Input: part model. Units: mm. Frame: model coordinates. A direction names the side the tool comes from. Round coordinates to 2 decimals unless told otherwise and drop trailing zeros. Loops run counter-clockwise (first coordinate to the right, second up) from the corner with the lowest first, then second, coordinate; pieces in that order, holes last. Notation, with made-up numbers: M 66,-17.75 L 77,-17.75 A5 ccw 77,-12.75 Z; hole C -1.5,29.5 d5. An arc over 180 degrees is marked long. Return JSON: item names as keys, results as strings. Group by question number.
1) Mould query, pull axis X, two halves, no side actions, for faces 1 (the face through (-8.577, 2.348, -103.456)), 2 (the face through (-217, 4.762, -61)), 3 (the face through (0, 7, -48)). Classes: +X half, -X half, draft (parallel to the pull), parting line (faces both ways), or undercut.
2) Section A-A (z = -84.5). Output: boundary loops of the cut face in (x, y), plus the area to 3 significant figures.
3) Contact query for flat-ended pins moving along their axis: P1, Ø10, axis at x = -52.5, y = 7, coming from the +Z side; P2, Ø15, axis at x = -119, y = 34, coming from the -Z side; P3, Ø4.5, axis at x = -298, y = 7.5, coming from the -Z side; P4, Ø1, axis at x = -162, y = 12, coming from the -Z side. Output: stop coordinate, or through.
4) Access query for faces 4 (the face through (-219, 4.762, -9)), 5 (the face through (-219, 9.538, -40)), 6 (the face through (-431.8, 7, -44)), 7 (the face through (-423.43, 2.348, -103.654)). Directions: +Z, -Z, +X, -X, +Y, -Y. A direction counts if a zero-diameter tool reaches every point of the face in a straight line with its end or side. Return the directions, or none.
5) Section C-C (y = 20). Output: boundary loops of the cut face in (x, z), plus the area to 3 significant figures.
6) Section B-B (x = -78.5). Output: boundary loops of the cut face in (y, z), plus the area to 3 significant figures.
7) Material intervals for line 1 (Y direction, x = -396.5, z = -32.5); line 2 (Z direction, x = -53.5, y = 5.5); line 3 (Z direction, x = -121.5, y = 35), sorted ascending. Write a range as from..to.
8) Section D-D (z = -67). Output: boundary loops of the cut face in (x, y), plus the area to 3 significant figures.
from build123d import *

# Parameters (mm, degrees)
F1_DEPTH = 4.7625
F3_DEPTH = 431.8


with BuildPart() as f1:
    # F0 (on Front) → F1 (new body)
    with BuildSketch(Plane.XZ):
        with BuildLine():
            Line((0, 0), (-215.9, 0))
            Line((-215.9, 0), (-431.8, 0))
            Line((-431.8, 0), (-431.8, -112.7125))
            Line((-431.8, -112.7125), (-427.228, -112.7125))
            ThreePointArc((-427.228, -112.7125), (-423.326818, -103.5544), (-414.02, -100.022664))
            Line((-414.02, -100.022664), (-414.02, -91.132664))
            ThreePointArc((-414.02, -91.132664), (-398.8091, -80.428959), (-394.97, -62.23))
            Line((-394.97, -62.23), (-215.9, -62.23))
            Line((-215.9, -62.23), (-36.83, -62.23))
            ThreePointArc((-36.83, -62.23), (-32.9909, -80.428959), (-17.78, -91.132664))
            Line((-17.78, -91.132664), (-17.78, -100.022664))
            ThreePointArc((-17.78, -100.022664), (-8.473182, -103.5544), (-4.572, -112.7125))
            Line((-4.572, -112.7125), (0, -112.7125))
            Line((0, -112.7125), (0, 0))
        make_face()
    extrude(amount=-F1_DEPTH)

    # F2 (on face) → F3 (join, through all)
    with BuildSketch(Plane(origin=(-431.8, 0, 0), x_dir=(0, -1, 0), z_dir=(-1, 0, 0))):
        with BuildLine():
            Line((-4.7625, -55.88), (-4.7625, -17.78))
            Line((-4.7625, -17.78), (-42.3545, -17.78))
            ThreePointArc((-42.3545, -17.78), (-42.71371, -17.92879), (-42.8625, -18.288))
            Line((-42.8625, -18.288), (-42.8625, -22.0345))
            ThreePointArc((-42.8625, -22.0345), (-42.71371, -22.39371), (-42.3545, -22.5425))
            Line((-42.3545, -22.5425), (-12.0777, -22.5425))
            ThreePointArc((-12.0777, -22.5425), (-10.281649, -23.286449), (-9.5377, -25.0825))
            Line((-9.5377, -25.0825), (-9.5377, -55.372))
            ThreePointArc((-9.5377, -55.372), (-9.38891, -55.73121), (-9.0297, -55.88))
            Line((-9.0297, -55.88), (-4.7625, -55.88))
        make_face()
    extrude(amount=-F3_DEPTH)


solid = f1.part
Returned:
{
 "1": {"face 1": "undercut", "face 2": "draft", "face 3": "+X half"},
 "2": {"outline": "M -431.8,0 L -402.15,0 L -402.15,4.76 L -431.8,4.76 Z; M -29.65,0 L 0,0 L 0,4.76 L -29.65,4.76 Z", "area": "282 mm^2"},
 "3": {"P1": "stops at z = 0", "P2": "stops at z = -22.54", "P3": "stops at z = -55.88", "P4": "stops at z = -22.61"},
 "4": {"face 4": "+Z, +X, -X, +Y", "face 5": "-Z, +X, -X, +Y", "face 6": "+Z, -Z, -X, +Y, -Y", "face 7": "-Z, +Y, -Y"},
 "5": {"outline": "M -431.8,-22.54 L 0,-22.54 L 0,-17.78 L -431.8,-17.78 Z", "area": "2,060 mm^2"},
 "6": {"outline": "M 0,-62.23 L 4.76,-62.23 L 4.76,-55.88 L 9.03,-55.88 A0.51 ccw 9.54,-55.37 L 9.54,-25.08 A2.54 cw 12.08,-22.54 L 42.35,-22.54 A0.51 ccw 42.86,-22.03 L 42.86,-18.29 A0.51 ccw 42.35,-17.78 L 4.76,-17.78 L 4.76,0 L 0,0 Z", "area": "638 mm^2"},
 "7": {"line 1": "y = 0..9.54", "line 2": "z = -55.88..-17.78", "line 3": "z = -22.54..-17.78"},
 "8": {"outline": "M -431.8,0 L -394.62,0 L -394.62,4.76 L -431.8,4.76 Z; M -37.18,0 L 0,0 L 0,4.76 L -37.18,4.76 Z", "area": "354 mm^2"}
}
